For this review, take the finished solid that the model builds, in its own axes (mm). Face numbers are marked on the shaded views. Coordinates: 2 decimals unless noted, no trailing zeros. Answer as a JSON object with one key per item and string values. Group by question number.
Item 1: Mouldability with a two-part tool opening along X and no side actions: class the marked faces 1 and 2 as +X half, -X half, draft (parallel to the pull), parting line (faces both ways), or undercut.
Item 2: Insertion check: pin 1 (4 mm diameter, centred on x = -9, z = 3, fed in from +Y); pin 2 (1 mm diameter, centred on x = 1.5, y = -11, fed in from -Z); pin 3 (2.5 mm diameter, centred on x = 0, y = 0, fed in from +Z); pin 4 (6 mm diameter, centred on y = 11, z = 7, fed in from +X). Each pin has a flat end and moves straight along its axis. Give the tip position at first contact, or say it passes through.
Item 3: Wall thickness on L1, parallel to Y at x = 0, z = 2.2; L2, parallel to Z at x = -6, y = -11; L3, parallel to X at y = 1.5, z = 4: over which ranges is each line inside the solid? List them lowest first. Write a range as from..to.
from build123d import *

# Parameters (mm, degrees)
ESQUISSE1_R             = 1
BOSS_EXTRU_1_DEPTH      = 20
ESQUISSE2_R             = 13
ESQUISSE2_R_2           = 3
ENL_V_MAT_EXTRU_1_DEPTH = 18
ESQUISSE3_R             = 3
ENL_V_MAT_EXTRU_2_DEPTH = 15


with BuildPart() as part:
    # Esquisse1 → Boss.-Extru.1 (new body)
    with BuildSketch(Plane.XY):
        Polygon((12.738384473, -7.436132127), (12.644521362, -6.571040977), (12.819850246, -6.222052689), (13.569932991, -5.780953088), (13.368385348, -4.934447607), (13.498591881, -4.56623666), (14.18747556, -4.034604965), (13.881421911, -3.22003505), (13.964452658, -2.838408351), (14.581273164, -2.224628712), (14.175540158, -1.454840618), (14.210085674, -1.065816647), (14.74511538, -0.379568735), (14.246101669, 0.333297521), (14.231617151, 0.723583623), (14.676418318, 1.471477268), (14.091993646, 2.116179358), (14.028707524, 2.501572546), (14.376265372, 3.299317195), (13.715646465, 3.865687783), (13.604556799, 4.240110176), (13.849390133, 5.075124919), (13.122995347, 5.554232002), (12.965854086, 5.911778736), (13.104101738, 6.770894891), (12.323386752, 7.155182664), (12.122672109, 7.490215013), (12.152153831, 8.359883807), (11.329430986, 8.643291822), (11.088308351, 8.950526125), (11.008559199, 9.81703236), (10.156803327, 9.995091104), (9.879075346, 10.269682094), (9.691353012, 11.119360449), (8.823996811, 11.189261829), (8.514043422, 11.426879041), (8.221308398, 12.246329582), (7.352030594, 12.206971211), (7.014739946, 12.403867279), (6.62160884, 13.180166781), (5.764118463, 13.032169365), (5.404809832, 13.185239121), (4.917482555, 13.906144876), (4.08530274, 13.651842422), (3.709642638, 13.758671865), (3.135804633, 14.41281476), (2.342059353, 14.05621777), (1.955972163, 14.115122135), (1.304673198, 14.692185945), (0.561880291, 14.238918166), (0.171454839, 14.248968497), (-0.547033712, 14.739852581), (-1.227159959, 14.197062317), (-1.61576643, 14.158100114), (-2.390113575, 14.555062937), (-2.996847164, 13.931310314), (-3.377506098, 13.843950035), (-4.195499918, 14.140731255), (-4.719272298, 13.445853226), (-5.085980477, 13.311472593), (-5.934720721, 13.503391795), (-6.367271689, 12.748347), (-6.714245905, 12.569065277), (-7.580347433, 12.653095779), (-7.914855402, 11.849791726), (-8.236623665, 11.628436292), (-9.106427538, 11.603252884), (-9.337617118, 10.764358158), (-9.629104949, 10.504419922), (-10.488893841, 10.37041976), (-10.613119033, 9.509164232), (-10.869729496, 9.214742573), (-11.705944022, 8.974038921), (-11.721245721, 8.104005105), (-11.938931915, 7.77974323), (-12.738384473, 7.436132127), (-12.644521362, 6.571040977), (-12.819850246, 6.222052689), (-13.569932991, 5.780953088), (-13.368385348, 4.934447607), (-13.498591881, 4.56623666), (-14.18747556, 4.034604965), (-13.881421911, 3.22003505), (-13.964452658, 2.838408351), (-14.581273164, 2.224628712), (-14.175540158, 1.454840618), (-14.210085674, 1.065816647), (-14.74511538, 0.379568735), (-14.246101669, -0.333297521), (-14.231617151, -0.723583623), (-14.676418318, -1.471477268), (-14.091993646, -2.116179358), (-14.028707524, -2.501572546), (-14.376265372, -3.299317195), (-13.715646465, -3.865687783), (-13.604556799, -4.240110176), (-13.849390133, -5.075124919), (-13.122995347, -5.554232002), (-12.965854086, -5.911778736), (-13.104101738, -6.770894891), (-12.323386752, -7.155182664), (-12.122672109, -7.490215013), (-12.152153831, -8.359883807), (-11.329430986, -8.643291822), (-11.088308351, -8.950526125), (-11.008559199, -9.81703236), (-10.156803327, -9.995091104), (-9.879075346, -10.269682094), (-9.691353012, -11.119360449), (-8.823996811, -11.189261829), (-8.514043422, -11.426879041), (-8.221308398, -12.246329582), (-7.352030594, -12.206971211), (-7.014739946, -12.403867279), (-6.62160884, -13.180166781), (-5.764118463, -13.032169365), (-5.404809832, -13.185239121), (-4.917482555, -13.906144876), (-4.08530274, -13.651842422), (-3.709642638, -13.758671865), (-3.135804633, -14.41281476), (-2.342059353, -14.05621777), (-1.955972163, -14.115122135), (-1.304673198, -14.692185945), (-0.561880291, -14.238918166), (-0.171454839, -14.248968497), (0.547033712, -14.739852581), (1.227159959, -14.197062317), (1.61576643, -14.158100114), (2.390113575, -14.555062937), (2.996847164, -13.931310314), (3.377506098, -13.843950035), (4.195499918, -14.140731255), (4.719272298, -13.445853226), (5.085980477, -13.311472593), (5.934720721, -13.503391795), (6.367271689, -12.748347), (6.714245905, -12.569065277), (7.580347433, -12.653095779), (7.914855402, -11.849791726), (8.236623665, -11.628436292), (9.106427538, -11.603252884), (9.337617118, -10.764358158), (9.629104949, -10.504419922), (10.488893841, -10.37041976), (10.613119033, -9.509164232), (10.869729496, -9.214742573), (11.705944022, -8.974038921), (11.721245721, -8.104005105), (11.938931915, -7.77974323), align=None)
        Circle(ESQUISSE1_R, mode=Mode.SUBTRACT)
    extrude(amount=BOSS_EXTRU_1_DEPTH)

    # Esquisse2 → Enlèv. mat.-Extru.1 (cut)
    with BuildSketch(Plane.XY.offset(20)):
        Circle(ESQUISSE2_R)
        Circle(ESQUISSE2_R_2, mode=Mode.SUBTRACT)
    extrude(amount=-ENL_V_MAT_EXTRU_1_DEPTH, mode=Mode.SUBTRACT)

    # Esquisse3 → Enlèv. mat.-Extru.2 (cut)
    with BuildSketch(Plane.XY.offset(20)):
        Circle(ESQUISSE3_R)
    extrude(amount=-ENL_V_MAT_EXTRU_2_DEPTH, mode=Mode.SUBTRACT)


solid = part.part
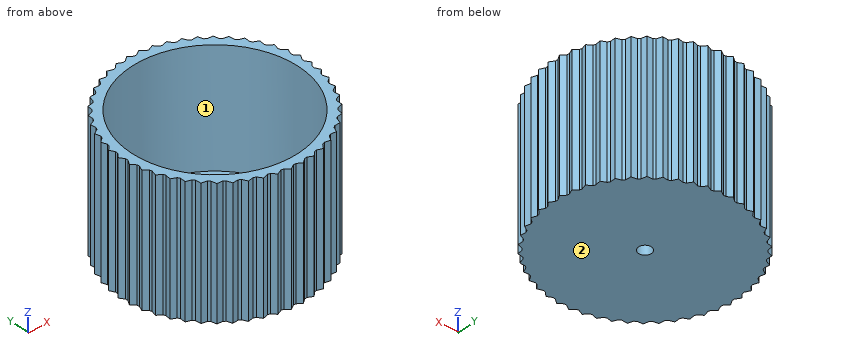
From the geometry:
{
 "1": {"face 1": "undercut", "face 2": "draft"},
 "2": {"pin 1": "stops at y = 12.65", "pin 2": "stops at z = 0", "pin 3": "stops at z = 5", "pin 4": "stops at x = 12.15"},
 "3": {"L1": "y = -14.37..-13, -3..-1, 1..3, 13..14.37", "L2": "z = 0..2", "L3": "x = -14.2..-12.91, -2.6..2.6, 12.91..14.65"}
}
